CAD build for the part. Positions are in the model's coordinates, mm. A direction names the side the tool comes from. Coordinates: 2 decimals unless noted, no trailing zeros. Loops run counter-clockwise (first coordinate to the right, second up) from the corner with the lowest first, then second, coordinate; pieces in that order, holes last.
1) Saw through at A-A, the plane y = -4.5. Write the cut outline in (x, z), and give its area (3 significant figures).
2) Wall check: line 1 along X through (y, z) = (8, 63.5); line 2 along Z through (x, y) = (-14, -51). Give the ranges that are in metal, low to high.
3) Saw through at C-C, the plane y = -44. Write the cut outline in (x, z), and give its area (3 significant figures).
4) Which spindle directions (+Z, -Z, +X, -X, +Y, -Y) get a long thin tool onto all of the face, cutting with end or side? Do faces 4 (the flat face through (-44, -1, 94)), 5 (the flat face through (-43, -1, 49)), 6 (the flat face through (6, -29, 2)). Say none if no direction does.
5) Pin check, flat tips, straight feed: pin 1 Ø1.5 at (y, z) = (-2, 2) entering from -X; pin 2 Ø6 at (x, y) = (-30, -3) entering from +Z; pin 3 Ø10 at (y, z) = (56, 46) entering from +X. Stop position of each tip, or through.
6) Saw through at B-B, the plane x = 14. Write the cut outline in (y, z).
7) Saw through at D-D, the plane z = 20. Write the cut outline in (x, y), and give its area (3 significant figures).
8) Two-plate mould, pull along X, no slides. Class faces 1 (the flat face through (46, -1, 1)), 2 (the flat face through (-46, -1, 50)), 3 (the flat face through (41, 18, 2)): +X half, -X half, draft (parallel to the pull), parting line (faces both ways), or undercut.
Autodesk Inventor part; units mm, degrees
ref_plane "YZ Plane" through (0, 0, 0) normal (1, 0, 0) x (0, 1, 0)
ref_plane "XZ Plane" through (0, 0, 0) normal (0, 1, 0) x (-1, 0, 0)
ref_plane "XY Plane" through (0, 0, 0) normal (0, 0, 1) x (1, 0, 0)
sketch "Sketch1" plane through (0, 0, 0) normal (0, 0, 1) x (1, 0, 0)
  line L0 (-46, -75) -> (46, -75)
  line L1 (46, -75) -> (46, 75)
  line L2 (46, 75) -> (-46, 75)
  line L3 (-46, 75) -> (-46, -75)
  line L4 (-46, -75) -> (46, 75) construction
  line L5 (46, -75) -> (-46, 75) construction
  point P0 (0, 0)
  dimension "d154" = 92
  dimension "d155" = 150
extrude "Plate5" add sketch "Sketch1" along normal blind 3
sketch "Sketch7" plane through (-43, -75, 0) normal (-1, 0, 0) x (0, -1, 0)
  line L0 (-150, 0) -> (0, 0)
  line L1 (0, 0) -> (0, 94)
  line L2 (0, 94) -> (-150, 94)
  line L3 (-150, 94) -> (-150, 0)
edge flange "Flange3" height 94 angle 90 thickness 3 bend radius 2.75 thickness toward (-1, 0, 0) relief round relief width 3 relief depth 1.5 edges at (-46, 0, 3) wall of the first edge with corners at (-43, 75, 0) (-43, -75, 0) (-43, -75, 94) (-43, 75, 94)
bend "Bend3"
corner "Corner3"
sketch "Sketch8" plane through (0, 0, 3) normal (0, 0, 1) x (1, 0, 0)
  line L0 (46, 75) -> (46, -75)
  line L1 (-40.25, 75) -> (46, 75)
  line L2 (41, 67) -> (-28, 67)
  line L3 (-28, 67) -> (-28, -29)
  line L4 (-28, -29) -> (41, -29)
  line L5 (41, -29) -> (41, 67)
  line L6 (41, 67) -> (-28, -29) construction
  line L7 (-28, 67) -> (41, -29) construction
  line L8 (-40.25, 75) -> (-43, 75)
  point P0 (0, 0)
  point P1 (6.5, 19)
  point P2 (2.875, 75)
  point P3 (-41.625, 75)
  dimension "d167" = 69
  dimension "d168" = 96
  dimension "d169" = 8
  dimension "d174" = 13.625
  dimension "d175" = 5
extrude "Cut1" cut sketch "Sketch8" against normal blind 3
properties part number "PNS 752 FDS 1200 FLANGE 2" material "Stainless Steel"
Data:
1. outline: (-46, 5.75) arc R5.75 ccw to (-40.25, 0) - (-28, 0) - (-28, 3) - (-40.25, 3) arc R2.75 cw to (-43, 5.75) - (-43, 94) - (-46, 94) - close; (41, 0) - (46, 0) - (46, 3) - (41, 3) - close
1. area: 337 mm2
2. line 1: x = -46 to -43
2. line 2: z = 0 to 3
3. outline: (-46, 5.75) arc R5.75 ccw to (-40.25, 0) - (46, 0) - (46, 3) - (-40.25, 3) arc R2.75 cw to (-43, 5.75) - (-43, 94) - (-46, 94) - close
3. area: 544 mm2
4. face 4: +Z, +X, -X, +Y, -Y
4. face 5: +Z, +X, +Y, -Y
4. face 6: +Z, -Z
5. pin 1: stops at x = -45.16
5. pin 2: stops at z = 3
5. pin 3: stops at x = -43
6. outline: (-75, 0) - (-29, 0) - (-29, 3) - (-75, 3) - close; (67, 0) - (75, 0) - (75, 3) - (67, 3) - close
7. outline: (-46, -75) - (-43, -75) - (-43, 75) - (-46, 75) - close
7. area: 450 mm2
8. face 1: +X half
8. face 2: -X half
8. face 3: undercut
